Verification items for the finished model (mm, model axes). Coordinates: 2 decimals unless noted, no trailing zeros. Order: outer loops, then holes, each group sorted by start corner. A loop starts at its lowest first (then second) coordinate and runs counter-clockwise, first axis right, second up. Notation, with made-up numbers: M 72,60 L 109,60 A17 ccw 109,77 Z; hole C -5,86 d10. An arc over 180 degrees is marked long. Return JSON: item names as keys, results as strings.
```python
from build123d import *

# Parameters (mm, degrees)
SKETCH1_R           = 4.5
BOSS_EXTRUDE1_DEPTH = 10


with BuildPart() as part:
    # Sketch1 → Boss-Extrude1 (new body)
    with BuildSketch(Plane(origin=(0, 0, 0), x_dir=(1, 0, 0), z_dir=(0, 1, 0))):
        Polygon((0, 0), (-200, 0), (-200, 100), (-170, 100), (-170, 30), (-30, 30), (-30, 100), (0, 100), align=None)
        with Locations((-15, 80)):
            Circle(SKETCH1_R, mode=Mode.SUBTRACT)
        with Locations((-15, 45)):
            Circle(SKETCH1_R, mode=Mode.SUBTRACT)
        with Locations((-130, 15)):
            Circle(SKETCH1_R, mode=Mode.SUBTRACT)
        with Locations((-70, 15)):
            Circle(SKETCH1_R, mode=Mode.SUBTRACT)
        with Locations((-185, 80)):
            Circle(SKETCH1_R, mode=Mode.SUBTRACT)
        with Locations((-185, 45)):
            Circle(SKETCH1_R, mode=Mode.SUBTRACT)
    extrude(amount=BOSS_EXTRUDE1_DEPTH)


solid = part.part
```
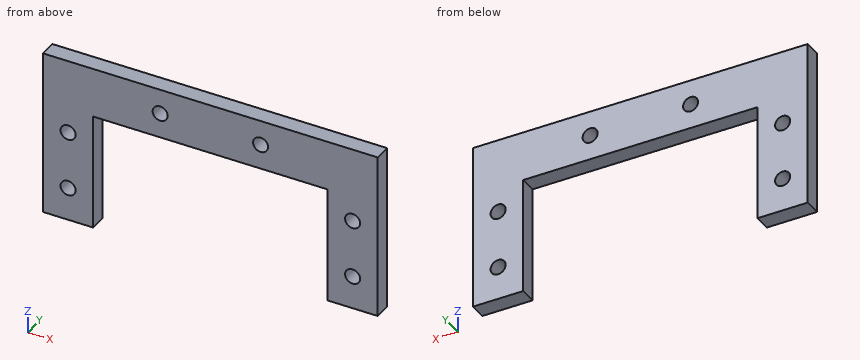
Q1. Cross-section at C-C, the plane x = -70. Record the boundary of the cut face in (y, z).
Values:
{"outline": "M 0,-30 L 10,-30 L 10,-19.5 L 0,-19.5 Z; M 0,-10.5 L 10,-10.5 L 10,0 L 0,0 Z"}
Q2. Cross-section at D-D, the plane y = 5.5. Record the boundary of the cut face in (x, z).
Values:
{"outline": "M -200,-100 L -170,-100 L -170,-30 L -30,-30 L -30,-100 L 0,-100 L 0,0 L -200,0 Z; hole C -185,-80 d9; hole C -185,-45 d9; hole C -130,-15 d9; hole C -70,-15 d9; hole C -15,-80 d9; hole C -15,-45 d9"}
Q3. Material ranges on line 1 along X through (y, z) = (4.75, -45); line 2 along X through (y, z) = (4.75, -66); line 3 along X through (y, z) = (8, -19), recorded low to high.
Values:
{"line 1": "-200 to -189.5, -180.5 to -170, -30 to -19.5, -10.5 to 0", "line 2": "-200 to -170, -30 to 0", "line 3": "-200 to -132.06, -127.94 to -72.06, -67.94 to 0"}
Q4. Cross-section at B-B, the plane z = -80. Record the boundary of the cut face in (x, y), and give its area (3 significant figures).
Values:
{"outline": "M -200,0 L -189.5,0 L -189.5,10 L -200,10 Z; M -180.5,0 L -170,0 L -170,10 L -180.5,10 Z; M -30,0 L -19.5,0 L -19.5,10 L -30,10 Z; M -10.5,0 L 0,0 L 0,10 L -10.5,10 Z", "area": "420 mm^2"}
Q5. Go/stop test with flat-tipped pins: pin 1 (10.5 mm diameter, centred on x = -15, z = -80, fed in from +Y); pin 2 (5 mm diameter, centred on x = -96, y = 4.5, fed in from -Z). Record where each tip stops, or that it passes through.
Values:
{"pin 1": "y = 10", "pin 2": "z = -30"}
Q6. Cross-section at A-A, the plane z = -15. Record the boundary of the cut face in (x, y), and give its area (3 significant figures).
Values:
{"outline": "M -200,0 L -134.5,0 L -134.5,10 L -200,10 Z; M -125.5,0 L -74.5,0 L -74.5,10 L -125.5,10 Z; M -65.5,0 L 0,0 L 0,10 L -65.5,10 Z", "area": "1,820 mm^2"}
